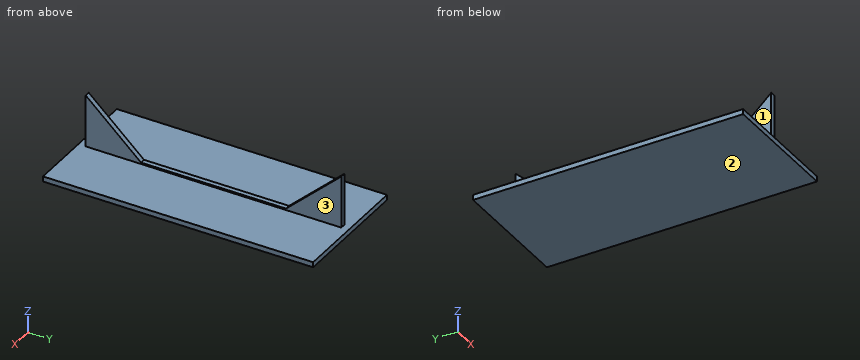
from build123d import *

# Parameters (mm, degrees)
SKICA1_W                 = 24
SKICA1_H                 = 51.8
P_IDAT_VYSUNUT_M2_DEPTH  = 1
SKICA2_W                 = 0.980102229
SKICA2_H                 = 51.8
P_IDAT_VYSUNUT_M3_DEPTH  = 0.28
SKICA3_W                 = 0.980102229
SKICA3_H                 = 12
P_IDAT_VYSUNUT_M5_DEPTH  = 11
ODEBRAT_VYSUNUT_M2_DEPTH = 11
ODEBRAT_VYSUNUT_M3_DEPTH = 11
SKICA9_W                 = 12.041997339
SKICA9_H                 = 1.4
ODEBRAT_VYSUNUT_M4_DEPTH = 11
SKICA10_W                = 11.638115032
SKICA10_H                = 1.404604082
ODEBRAT_VYSUNUT_M5_DEPTH = 11


with BuildPart() as part:
    # Skica1 → Přidat vysunutím2 (new body)
    with BuildSketch(Plane.XY):
        Rectangle(SKICA1_W, SKICA1_H)
    extrude(amount=P_IDAT_VYSUNUT_M2_DEPTH)

    # Skica2 → Přidat vysunutím3 (add)
    with BuildSketch(Plane.XY.offset(1)):
        with Locations((5.1115e-05, 0)):
            Rectangle(SKICA2_W, SKICA2_H)
    extrude(amount=P_IDAT_VYSUNUT_M3_DEPTH)

    # Skica3 → Přidat vysunutím5 (add)
    with BuildSketch(Plane.XY.offset(1.28)):
        with Locations((5.1115e-05, 19.9)):
            Rectangle(SKICA3_W, SKICA3_H)
        with Locations((5.1115e-05, -19.9)):
            Rectangle(SKICA3_W, SKICA3_H)
    extrude(amount=P_IDAT_VYSUNUT_M5_DEPTH)

    # Skica6 → Odebrat vysunutím2 (cut)
    with BuildSketch(Plane(origin=(0.490102229, 0, 0), x_dir=(0, 0, -1), z_dir=(1, 0, 0))):
        Polygon((-12.28, 25.9), (-12.28, 13.9), (-1.28, 13.9), align=None)
    extrude(amount=-ODEBRAT_VYSUNUT_M2_DEPTH, mode=Mode.SUBTRACT)

    # Skica7 → Odebrat vysunutím3 (cut)
    with BuildSketch(Plane.ZY.offset(0.49)):
        Polygon((12.28, -13.9), (12.28, -25.9), (1.28, -13.9), align=None)
    extrude(amount=-ODEBRAT_VYSUNUT_M3_DEPTH, mode=Mode.SUBTRACT)

    # Skica9 → Odebrat vysunutím4 (cut)
    with BuildSketch(Plane.ZY.offset(0.49)):
        with Locations((7.02099867, 25.2)):
            Rectangle(SKICA9_W, SKICA9_H)
    extrude(amount=-ODEBRAT_VYSUNUT_M4_DEPTH, mode=Mode.SUBTRACT)

    # Skica10 → Odebrat vysunutím5 (cut)
    with BuildSketch(Plane.ZY.offset(0.49)):
        with Locations((6.819057516, -25.197697959)):
            Rectangle(SKICA10_W, SKICA10_H)
    extrude(amount=-ODEBRAT_VYSUNUT_M5_DEPTH, mode=Mode.SUBTRACT)


solid = part.part
Design review of the part built by this model. Coordinates are the model's own, in mm. Face numbers are marked on the shaded views. A direction names the side the tool comes from. Round coordinates to 2 decimals unless told otherwise and drop trailing zeros. Write each loop counter-clockwise with the first axis right and the second up, starting at its lowest first coordinate (ties: lowest second). Pieces come first, ordered by that corner, then holes.
Item 1: Consider section B-B on z = 3.5. Give the boundary of the cut face in (x, y), and give its area (3 significant figures).
Item 2: For pin 1 Ø1.1 at (x, y) = (0, 1.5) entering from +Z; pin 2 Ø5 at (x, z) = (6, 3) entering from -Y; pin 3 Ø6 at (y, z) = (20.5, 9.5) entering from +X; pin 4 Ø1.5 at (x, y) = (-7, -18) entering from +Z, all flat-tipped, find the tip position at first contact; note any pin that passes through.
Item 3: Consider section C-C on x = -5.75. Give the boundary of the cut face in (y, z).
Item 4: For the marked faces 1, 2 and 3, list the 3-axis set-ups (+Z, -Z, +X, -X, +Y, -Y) from which the entire face can be reached by the end or side of a thin tool; tool diameter is ignored.
Item 5: Consider section D-D on z = 6. Give the boundary of the cut face in (x, y), and give its area (3 significant figures).
Item 6: Consider section A-A on y = 10. Give the boundary of the cut face in (x, z), and give its area (3 significant figures).
Item 7: Wall thickness on L1, parallel to X at y = 22, z = 6; L2, parallel to Z at x = 1.25, y = 18.5; L3, parallel to Z at x = -0.25, y = -22 (3 decimals): over which ranges is each line inside the solid? List them lowest first.
Check values:
1. outline: (-0.49, -24.5) - (0.49, -24.5) - (0.49, -16.32) - (-0.49, -16.32) - close; (-0.49, 16.32) - (0.49, 16.32) - (0.49, 24.5) - (-0.49, 24.5) - close
1. area: 16.0 mm2
2. pin 1: stops at z = 1.28
2. pin 2: stops at y = -25.9
2. pin 3: stops at x = 0.49
2. pin 4: stops at z = 1
3. outline: (-25.9, 0) - (25.9, 0) - (25.9, 1) - (-25.9, 1) - close
4. face 1: +Z, -X, +Y, -Y
4. face 2: -Z, +X, -X, +Y, -Y
4. face 3: +Z, +X, +Y, -Y
5. outline: (-0.49, -24.5) - (0.49, -24.5) - (0.49, -19.05) - (-0.49, -19.05) - close; (-0.49, 19.05) - (0.49, 19.05) - (0.49, 24.5) - (-0.49, 24.5) - close
5. area: 10.7 mm2
6. outline: (-12, 0) - (12, 0) - (12, 1) - (0.49, 1) - (0.49, 1.28) - (-0.49, 1.28) - (-0.49, 1) - (-12, 1) - close
6. area: 24.3 mm2
7. L1: x = -0.49 to 0.49
7. L2: z = 0 to 1
7. L3: z = 0 to 8.705
